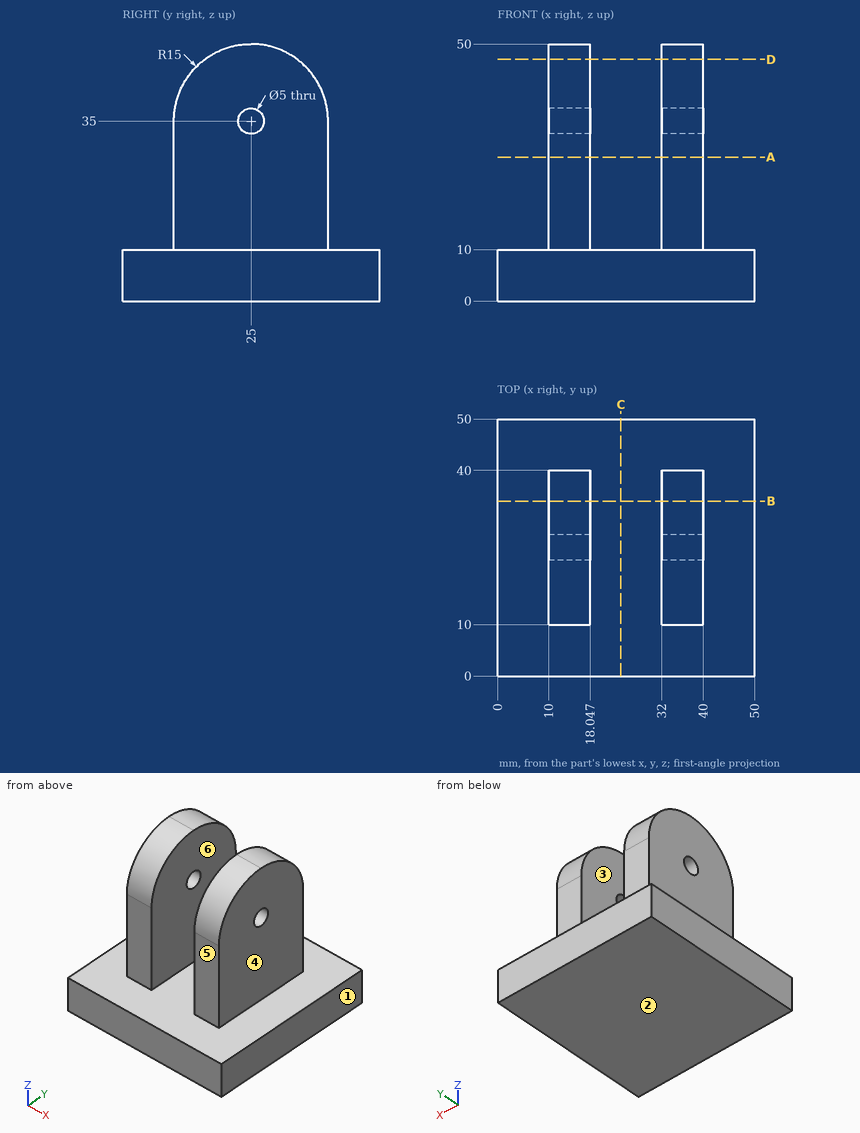
Geometry check sheet. Reference: drawing and pictorial views, mm from the part's lowest x, y, z. A direction names the side the tool comes from. Round coordinates to 2 decimals unless told otherwise and drop trailing zeros. Write each loop counter-clockwise with the first axis right and the second up, starting at its lowest first coordinate (ties: lowest second). Pieces come first, ordered by that corner, then holes. Notation, with made-up numbers: (75, 29) -> (128, 29) arc R20 ccw to (128, 44) -> close; hole circle Ø10 at (79, -31). An arc over 180 degrees is marked (long way). Put each result on its own line as item: value.
1) Thickness scan on probe 1 along X at (y, z) = (12.5, 26); probe 2 along Z at (x, y) = (35, 25); probe 3 along Z at (x, y) = (27, 29.5). Record the ranges inside material, lowest first. Write a range as from..to.
Recorded:
probe 1: x = 10..18.05, 32..40
probe 2: z = 0..32.5, 37.5..50
probe 3: z = 0..10
2) Cross-section at C-C, the plane x = 24. Enter the section's corners in (y, z), plus the area to 3 significant figures.
Recorded:
outline: (0, 0) -> (50, 0) -> (50, 10) -> (0, 10) -> close
area: 500 mm2
3) Release check for a two-part mould opening along X. For the marked faces 1, 2 and 3 record: pulls with the +X half, pulls with the -X half, needs draft (parallel to the pull), parting line crosses it, or undercut.
Recorded:
face 1: pulls with the +X half
face 2: needs draft
face 3: undercut
4) Cross-section at B-B, the plane y = 34. Enter the section's corners in (x, z), plus the area to 3 significant figures.
Recorded:
outline: (0, 0) -> (50, 0) -> (50, 10) -> (40, 10) -> (40, 47) -> (32, 47) -> (32, 10) -> (18.05, 10) -> (18.05, 47) -> (10, 47) -> (10, 10) -> (0, 10) -> close
area: 1,090 mm2
5) Access from +Z, -Z, +X, -X, +Y, -Y to the whole of each face (thin tool, end or side, straight path). Record for the marked faces 4, 5 and 6.
Recorded:
face 4: +Z, +X, +Y, -Y
face 5: +Z, +X, -X, -Y
face 6: +Z, +Y, -Y
6) Cross-section at D-D, the plane z = 47. Enter the section's corners in (x, y), plus the area to 3 significant figures.
Recorded:
outline: (10, 16) -> (18.05, 16) -> (18.05, 34) -> (10, 34) -> close; (32, 16) -> (40, 16) -> (40, 34) -> (32, 34) -> close
area: 289 mm2
7) Depth check by flat-ended pin: P1, Ø4, axis at x = 38, z = 19, coming from the +Y side; P2, Ø10, axis at y = 25.5, z = 37.5, coming from the +X side; P3, Ø12, axis at x = 16, y = 24, coming from the -Z side; P4, Ø9, axis at y = 20, z = 31.5, coming from the -X side. Enter the tip coordinate at first touch or a pass-through.
Recorded:
P1: stops at y = 40
P2: stops at x = 40
P3: stops at z = 0
P4: stops at x = 10
8) Cross-section at A-A, the plane z = 28. Enter the section's corners in (x, y).
Recorded:
outline: (10, 10) -> (18.05, 10) -> (18.05, 40) -> (10, 40) -> close; (32, 10) -> (40, 10) -> (40, 40) -> (32, 40) -> close
